from build123d import *

# Parameters (mm, degrees)
SKETCH1_W           = 33
SKETCH1_H           = 33
SKETCH1_R           = 2.75
BOSS_EXTRUDE1_DEPTH = 17
SKETCH2_W           = 25
SKETCH2_H           = 25
CUT_EXTRUDE2_DEPTH  = 14
SKETCH3_W           = 4
SKETCH3_H           = 3
CUT_EXTRUDE3_DEPTH  = 14
SKETCH4_W           = 15.227626713
SKETCH4_H           = 4
CUT_EXTRUDE4_DEPTH  = 14
SKETCH5_W           = 4
SKETCH5_H           = 9.93135505
CUT_EXTRUDE5_DEPTH  = 14
SKETCH6_W           = 27.732245768
SKETCH6_H           = 12.796931656
CUT_EXTRUDE6_DEPTH  = 14
SKETCH7_W           = 1
SKETCH7_H           = 6
BOSS_EXTRUDE2_DEPTH = 14
SKETCH8_W           = 4
SKETCH8_H           = 2
CUT_EXTRUDE7_DEPTH  = 14


with BuildPart() as part:
    # Sketch1 → Boss-Extrude1 (new body)
    with BuildSketch(Plane(origin=(0, 0, 0), x_dir=(1, 0, 0), z_dir=(0, 1, 0))):
        with Locations((-1.794117647, -1.647058824)):
            Rectangle(SKETCH1_W, SKETCH1_H)
        with Locations(Location((-1.794117647, -1.647058824, 0), (0, 0, 270))):
            Circle(SKETCH1_R, mode=Mode.SUBTRACT)
    extrude(amount=BOSS_EXTRUDE1_DEPTH)

    # Sketch2 → Cut-Extrude2 (cut)
    with BuildSketch(Plane(origin=(0, 17, 0), x_dir=(1, 0, 0), z_dir=(0, 1, 0))):
        with Locations((-1.794117647, -1.647058824)):
            Rectangle(SKETCH2_W, SKETCH2_H)
    extrude(amount=-CUT_EXTRUDE2_DEPTH, mode=Mode.SUBTRACT)

    # Sketch3 → Cut-Extrude3 (cut)
    with BuildSketch(Plane(origin=(0, 17, 0), x_dir=(1, 0, 0), z_dir=(0, 1, 0))):
        with Locations((12.705882353, 3.421586126)):
            Rectangle(SKETCH3_W, SKETCH3_H)
        with Locations((-16.294117647, 3.421586126)):
            Rectangle(SKETCH3_W, SKETCH3_H)
    extrude(amount=-CUT_EXTRUDE3_DEPTH, mode=Mode.SUBTRACT)

    # Sketch4 → Cut-Extrude4 (cut)
    with BuildSketch(Plane(origin=(0, 17, 0), x_dir=(1, 0, 0), z_dir=(0, 1, 0))):
        with Locations((3.092068996, 12.852941176)):
            Rectangle(SKETCH4_W, SKETCH4_H)
    extrude(amount=-CUT_EXTRUDE4_DEPTH, mode=Mode.SUBTRACT)

    # Sketch5 → Cut-Extrude5 (cut)
    with BuildSketch(Plane(origin=(0, 17, 0), x_dir=(1, 0, 0), z_dir=(0, 1, 0))):
        with Locations((12.705882353, 9.887263651)):
            Rectangle(SKETCH5_W, SKETCH5_H)
    extrude(amount=-CUT_EXTRUDE5_DEPTH, mode=Mode.SUBTRACT)

    # Sketch6 → Cut-Extrude6 (cut)
    with BuildSketch(Plane(origin=(0, 17, 0), x_dir=(1, 0, 0), z_dir=(0, 1, 0))):
        with Locations((-12.170590875, 9.919039286)):
            Rectangle(SKETCH6_W, SKETCH6_H)
    extrude(amount=-CUT_EXTRUDE6_DEPTH, mode=Mode.SUBTRACT)

    # Sketch7 → Boss-Extrude2 (add)
    with BuildSketch(Plane(origin=(0, 3, 0), x_dir=(1, 0, 0), z_dir=(0, 1, 0))):
        with Locations((15.205882353, -1.078413874)):
            Rectangle(SKETCH7_W, SKETCH7_H)
        with Locations((-18.794117647, -1.078413874)):
            Rectangle(SKETCH7_W, SKETCH7_H)
    extrude(amount=BOSS_EXTRUDE2_DEPTH)

    # Sketch8 → Cut-Extrude7 (cut)
    with BuildSketch(Plane(origin=(0, 17, 0), x_dir=(1, 0, 0), z_dir=(0, 1, 0))):
        with Locations((-16.294117647, -7.147058824)):
            Rectangle(SKETCH8_W, SKETCH8_H)
    extrude(amount=-CUT_EXTRUDE7_DEPTH, mode=Mode.SUBTRACT)


solid = part.part
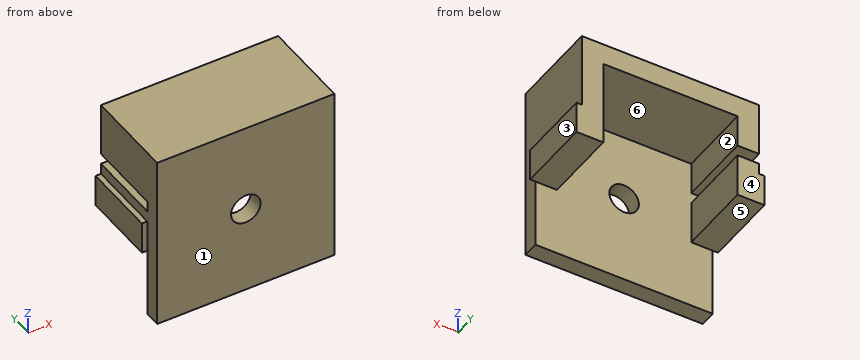
Read the model definition and answer for the solid it produces. Units are mm, in the model's axes. Face numbers are marked on the shaded views. A direction names the side the tool comes from. Give positions to 0.01 mm unless a question says otherwise; leave off trailing zeros. Loops run counter-clockwise (first coordinate to the right, second up) from the corner with the lowest first, then second, coordinate; pieces in that order, holes last. Notation, with made-up numbers: (72, 67) -> (77, 67) arc R8 cw to (77, 82) -> close; hole circle Ø9 at (50.5, 55). An arc over 180 degrees is marked (long way). Use a Markdown table: item, result.
Q1. Section A-A, the plane y = 13.25 is taken. Determine the outline of the cut face in (x, z).
Solved:
| item | result |
|---|---|
| outline | (-19.29, -1.92) -> (-14.29, -1.92) -> (-14.29, 6.15) -> (-18.29, 6.15) -> (-18.29, 4.08) -> (-19.29, 4.08) -> close; (-18.29, 8.15) -> (-14.29, 8.15) -> (-14.29, 14.15) -> (10.71, 14.15) -> (10.71, -1.92) -> (15.71, -1.92) -> (15.71, 4.08) -> (14.71, 4.08) -> (14.71, 18.15) -> (-18.29, 18.15) -> close |
Q2. Section D-D, the plane z = 10 is taken. Determine the outline of the cut face in (x, y), then the cut area to 3 significant figures.
Solved:
| item | result |
|---|---|
| outline | (-18.29, 0) -> (14.71, 0) -> (14.71, 17) -> (10.71, 17) -> (10.71, 3) -> (-14.29, 3) -> (-14.29, 17) -> (-18.29, 17) -> close |
| area | 211 mm^2 |
Q3. Each of these flat-tipped pins is pushed along its axis until it touches: pin 1 (3 mm diameter, centred on y = 11.5, z = 11, fed in from +X); pin 2 (2 mm diameter, centred on x = -16, y = 13, fed in from -Z); pin 3 (8 mm diameter, centred on x = 0, y = 8.5, fed in from -Z); pin 4 (4.5 mm diameter, centred on x = -1.79, z = 1.65, fed in from +Y). Where does it stop, or does it pass through?
Solved:
| item | result |
|---|---|
| pin 1 | stops at x = 14.71 |
| pin 2 | stops at z = -1.92 |
| pin 3 | stops at z = 14.15 |
| pin 4 | passes through |
Q4. Section C-C, the plane x = -5.5 is taken. Determine the outline of the cut face in (y, z).
Solved:
| item | result |
|---|---|
| outline | (0, -14.85) -> (3, -14.85) -> (3, 14.15) -> (17, 14.15) -> (17, 18.15) -> (0, 18.15) -> close |
Q5. Section B-B, the plane z = 2 is taken. Determine the outline of the cut face in (x, y).
Solved:
| item | result |
|---|---|
| outline | (-19.29, 3) -> (-18.29, 3) -> (-18.29, 0) -> (-4.52, 0) -> (-4.52, 3) -> (-14.29, 3) -> (-14.29, 17) -> (-19.29, 17) -> close; (0.93, 0) -> (14.71, 0) -> (14.71, 3) -> (15.71, 3) -> (15.71, 17) -> (10.71, 17) -> (10.71, 3) -> (0.93, 3) -> close |
Q6. Determine the mould class of the marked faces 1, 2 and 3 for opening direction X: pulls with the +X half, pulls with the -X half, needs draft (parallel to the pull), parting line crosses it, or undercut.
Solved:
| item | result |
|---|---|
| face 1 | needs draft |
| face 2 | undercut |
| face 3 | pulls with the +X half |
Q7. A tool of negligible diameter and unlimited length cuts with its end or side. For the marked faces 4, 5 and 6, from which of +Z, -Z, +X, -X, +Y, -Y can it reach the whole face along a straight path? Write none if from no direction.
Solved:
| item | result |
|---|---|
| face 4 | +Z, -Z, +X, -X, +Y |
| face 5 | -Z, +X, -X, +Y |
| face 6 | -Z, +Y |
Q8. Find the intervals of material crossed by line 1 along X through (y, z) = (6, 2.5); line 2 along Y through (x, z) = (-9.5, -4); line 3 along X through (y, z) = (3.75, 15), in increasing order.
Solved:
| item | result |
|---|---|
| line 1 | x = -19.29 to -14.29, 10.71 to 15.71 |
| line 2 | y = 0 to 3 |
| line 3 | x = -18.29 to 14.71 |
